```python
from build123d import *

# Parameters (mm, degrees)
SKETCH1_R           = 6.25
SKETCH1_R_2         = 1.75
BOSS_EXTRUDE1_DEPTH = 10


with BuildPart() as part:
    # Sketch1 → Boss-Extrude1 (new body)
    with BuildSketch(Plane.XY):
        with BuildLine():
            Line((40.062548905, 177), (43.062548905, 177))
            ThreePointArc((43.062548905, 177), (44.476762467, 176.414213562), (45.062548905, 175))
            Line((45.062548905, 175), (45.062548905, 139))
            ThreePointArc((45.062548905, 139), (45.648335342, 137.585786438), (47.062548905, 137))
            Line((47.062548905, 137), (112.937451095, 137))
            ThreePointArc((112.937451095, 137), (114.351664658, 137.585786438), (114.937451095, 139))
            Line((114.937451095, 139), (114.937451095, 175))
            ThreePointArc((114.937451095, 175), (115.523237533, 176.414213562), (116.937451095, 177))
            Line((116.937451095, 177), (120, 177))
            Line((120, 177), (152, 177))
            ThreePointArc((152, 177), (157.656854249, 174.656854249), (160, 169))
            Line((160, 169), (160, 0))
            Line((160, 0), (120, 0))
            Line((120, 0), (40, 0))
            Line((40, 0), (0, 0))
            Line((0, 0), (0, 169))
            ThreePointArc((0, 169), (2.343145751, 174.656854249), (8, 177))
            Line((8, 177), (40, 177))
            Line((40, 177), (40.062548905, 177))
        make_face()
        with Locations((20, 162)):
            Circle(SKETCH1_R, mode=Mode.SUBTRACT)
        with Locations((140, 162)):
            Circle(SKETCH1_R, mode=Mode.SUBTRACT)
        with Locations((4.328403696, 49)):
            Circle(SKETCH1_R_2, mode=Mode.SUBTRACT)
        with Locations((4.328403696, 29)):
            Circle(SKETCH1_R_2, mode=Mode.SUBTRACT)
        with Locations((36.371302772, 4.5)):
            Circle(SKETCH1_R_2, mode=Mode.SUBTRACT)
        with Locations((123.628697228, 4.5)):
            Circle(SKETCH1_R_2, mode=Mode.SUBTRACT)
        with Locations((155.671596304, 29)):
            Circle(SKETCH1_R_2, mode=Mode.SUBTRACT)
        with Locations((155.671596304, 49)):
            Circle(SKETCH1_R_2, mode=Mode.SUBTRACT)
    extrude(amount=BOSS_EXTRUDE1_DEPTH)


solid = part.part
```
CAD build for the part. Positions are in the model's coordinates, mm. A direction names the side the tool comes from. Round coordinates to 2 decimals unless told otherwise and drop trailing zeros. Write each loop counter-clockwise with the first axis right and the second up, starting at its lowest first coordinate (ties: lowest second). Pieces come first, ordered by that corner, then holes.
Item 1: Drill centre lines: L1, parallel to Y at x = 19.5, z = 1; L2, parallel to X at y = 145.5, z = 7.75; L3, parallel to Y at x = 65, z = 8. Where is each one in solid material? Low to high.
Filled in:
L1: y = 0 to 155.77, 168.23 to 177
L2: x = 0 to 45.06, 114.94 to 160
L3: y = 0 to 137
Item 2: Band-saw the part on B-B on x = 140. Write the cut outline in (y, z).
Filled in:
outline: (0, 0) - (155.75, 0) - (155.75, 10) - (0, 10) - close; (168.25, 0) - (177, 0) - (177, 10) - (168.25, 10) - close
Item 3: Tool access for faces 5 (the flat face through (114.937, 157, 5)), 6 (the cylindrical face through (2.281, 174.594, 4.93)): list every direction of +Z, -Z, +X, -X, +Y, -Y with a clear straight run to the whole face (end or side of a thin tool).
Filled in:
face 5: +Z, -Z, +Y
face 6: +Z, -Z, -X, +Y
Item 4: Band-saw the part on C-C on z = 7.5. Give the number of separate pieces and of enclosed holes in the cut face, then the cut area to 3 significant figures.
Filled in:
separate pieces: 1
enclosed holes: 8
area: 25,200 mm2
Item 5: Band-saw the part on A-A on y = 162. Write the cut outline in (x, z), then the cut area to 3 significant figures.
Filled in:
outline: (0, 0) - (13.75, 0) - (13.75, 10) - (0, 10) - close; (26.25, 0) - (45.06, 0) - (45.06, 10) - (26.25, 10) - close; (114.94, 0) - (133.75, 0) - (133.75, 10) - (114.94, 10) - close; (146.25, 0) - (160, 0) - (160, 10) - (146.25, 10) - close
area: 651 mm2
Item 6: Mould opens along Y. For faces 1 (the flat face through (25, 177, 5)), 2 (the flat face through (81, 0, 5)), 3 (the cylindrical face through (145.773, 159.606, 4.93)), 4 (the flat face through (81, 90, 0)) say: released by +Y, released by -Y, zero draft, split by the parting line, or undercut.
Filled in:
face 1: released by +Y
face 2: released by -Y
face 3: undercut
face 4: zero draft
Item 7: Band-saw the part on D-D on x = 104. Write the cut outline in (y, z), then the cut area to 3 significant figures.
Filled in:
outline: (0, 0) - (137, 0) - (137, 10) - (0, 10) - close
area: 1,370 mm2
Item 8: Drop flat-ended pins along their axis: pin 1 Ø1 at (x, z) = (106.5, 8) entering from +Y; pin 2 Ø3 at (x, y) = (123.63, 4.5) entering from -Z. Give the stop position or say it passes through.
Filled in:
pin 1: stops at y = 137
pin 2: passes through
